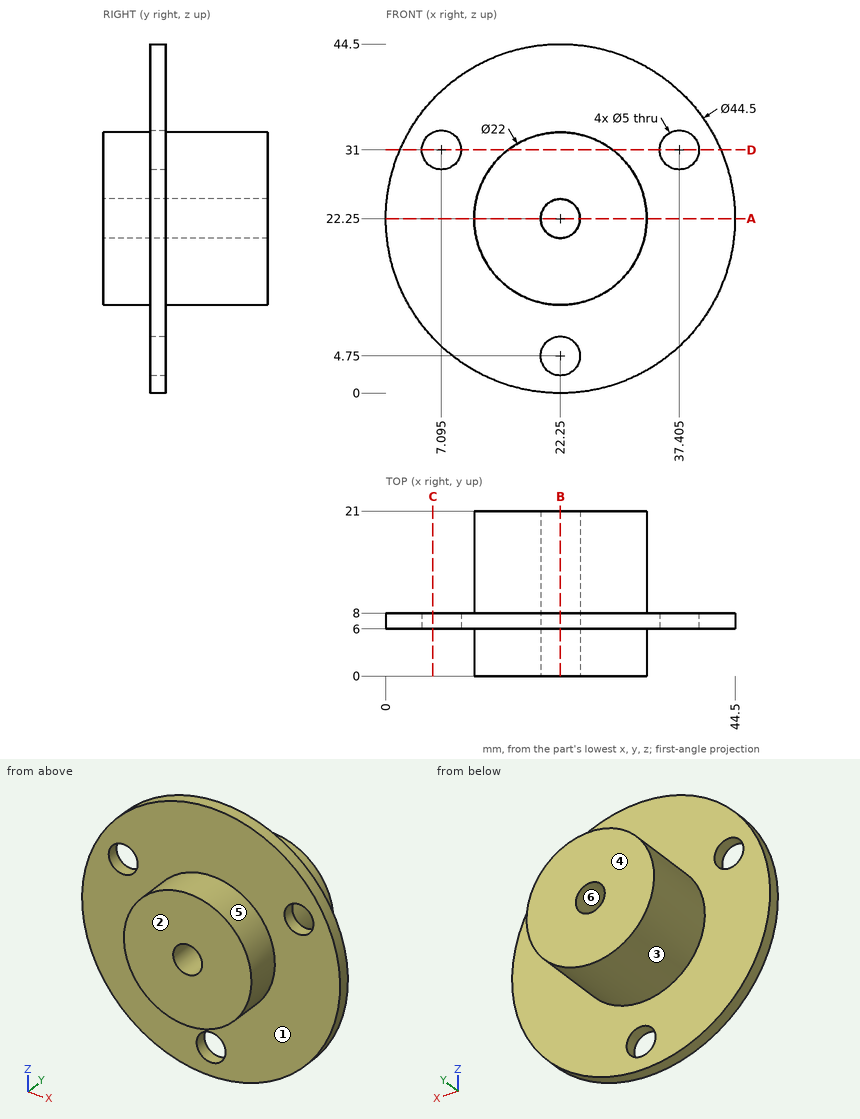
Study the drawing (mm; zero at the part's minimum x, y, z) and answer. A direction names the side the tool comes from. Give positions to 0.01 mm unless a question says otherwise; leave off trailing zeros. Order: outer loops, then holes, each group sorted by start corner. A loop starts at its lowest first (then second) coordinate and runs counter-clockwise, first axis right, second up.
1. The mould has two halves that part along Z. Classify the marked faces 4, 5 and 6: released by +Z, released by -Z, zero draft, split by the parting line, or undercut.
Result sheet:
face 4: zero draft
face 5: split by the parting line
face 6: undercut
2. Section D-D, the plane z = 31 is taken. Determine the outline of the cut face in (x, y) (1 decimal).
Result sheet:
outline: (1.8, 6) - (4.6, 6) - (4.6, 8) - (1.8, 8) - close; (9.6, 6) - (15.6, 6) - (15.6, 0) - (28.9, 0) - (28.9, 6) - (34.9, 6) - (34.9, 8) - (28.9, 8) - (28.9, 21) - (15.6, 21) - (15.6, 8) - (9.6, 8) - close; (39.9, 6) - (42.7, 6) - (42.7, 8) - (39.9, 8) - close
3. For the marked faces 1, 2 and 3, determine the directions among +Z, -Z, +X, -X, +Y, -Y from which every point of the face is accessible in a straight line to the end or side of a thin tool.
Result sheet:
face 1: -Y
face 2: +Z, -Z, +X, -X, -Y
face 3: +Y
4. Section B-B, the plane x = 22.25 is taken. Determine the outline of the cut face in (y, z), and give its area (3 significant figures).
Result sheet:
outline: (0, 11.25) - (6, 11.25) - (6, 7.25) - (8, 7.25) - (8, 11.25) - (21, 11.25) - (21, 19.75) - (0, 19.75) - close; (0, 24.75) - (21, 24.75) - (21, 33.25) - (8, 33.25) - (8, 44.5) - (6, 44.5) - (6, 33.25) - (0, 33.25) - close; (6, 0) - (8, 0) - (8, 2.25) - (6, 2.25) - close
area: 392 mm2
5. Section C-C, the plane x = 6 is taken. Determine the outline of the cut face in (y, z).
Result sheet:
outline: (6, 7.05) - (8, 7.05) - (8, 28.75) - (6, 28.75) - close; (6, 33.25) - (8, 33.25) - (8, 37.45) - (6, 37.45) - close
6. Each of these flat-tipped pins is pushed along its axis until it touches: P1, Ø3, axis at x = 33.5, y = 6.5, coming from the -Z side; P2, Ø8, axis at y = 11, z = 34.5, coming from the +X side; P3, Ø12, axis at y = 15.5, z = 19.5, coming from the -X side. Where does it stop, or does it pass through?
Result sheet:
P1: stops at z = 2.25
P2: stops at x = 42.32
P3: stops at x = 11.25
7. Straight lines are drawn through the part: L1, parallel to Z at x = 22, y = 13; L2, parallel to X at y = 6.6, z = 31 (1 decimal); L3, parallel to Y at x = 42, z = 22. For each, find the intervals that lie inside material, in ascending order.
Result sheet:
L1: z = 11.25 to 19.76, 24.74 to 33.25
L2: x = 1.8 to 4.6, 9.6 to 34.9, 39.9 to 42.7
L3: y = 6 to 8
8. Section A-A, the plane z = 22.25 is taken. Determine the outline of the cut face in (x, y).
Result sheet:
outline: (0, 6) - (11.25, 6) - (11.25, 0) - (19.75, 0) - (19.75, 21) - (11.25, 21) - (11.25, 8) - (0, 8) - close; (24.75, 0) - (33.25, 0) - (33.25, 6) - (44.5, 6) - (44.5, 8) - (33.25, 8) - (33.25, 21) - (24.75, 21) - close
